Design review of the part built by this model. Coordinates are the model's own, in mm. Face numbers are marked on the shaded views. Round coordinates to 2 decimals unless told otherwise and drop trailing zeros. Write each loop counter-clockwise with the first axis right and the second up, starting at its lowest first coordinate (ties: lowest second). Pieces come first, ordered by that corner, then holes. Notation, with made-up numbers: M 72.25,-21.5 L 129.25,-21.5 A19 cw 129.25,-11.5 Z; hole C 36,5 d11. An arc over 180 degrees is marked long. Use CSV: the item, a comma, the result in double quotes.
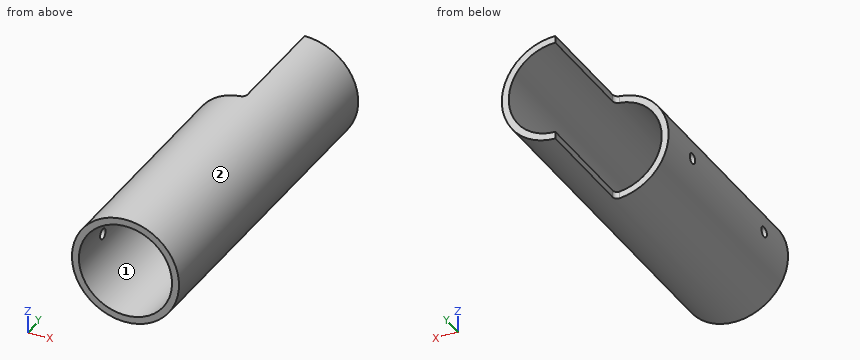
Autodesk Inventor part; units mm, degrees
ref_plane "YZ Plane" through (0, 0, 0) normal (1, 0, 0) x (0, 1, 0)
ref_plane "XZ Plane" through (0, 0, 0) normal (0, 1, 0) x (-1, 0, 0)
ref_plane "XY Plane" through (0, 0, 0) normal (0, 0, 1) x (1, 0, 0)
sketch "Sketch1" plane through (0, 0, 0) normal (0, 1, 0) x (-1, 0, 0)
  circle A0 centre (0, 0) radius 20
  circle A1 centre (0, 0) radius 23
  dimension "d0" = 40
  dimension "d1" = 3
extrude "Extrusion1" add sketch "Sketch1" along normal mid plane 150
sketch "Sketch2" plane through (0, 0, 0) normal (1, 0, 0) x (0, 1, 0)
  line L0 (-105, 0) -> (105, 0)
  line L1 (-75, 23) -> (-75, -23)
  point P0 (0, 0)
  point P1 (5, 0)
  point P2 (-55, 0)
  dimension "d4" = 60
  dimension "d5" = 20
hole "Hole1" at (0, 5, 0) at (0, -55, 0) direction (-1, 0, 0) diameter 4.5 end through all
sketch "Sketch3" plane through (0, 0, 0) normal (0, 0, 1) x (1, 0, 0)
  line L0 (23, 75) -> (-23, 75)
  line L1 (-23, -75) -> (-23, 75)
  line L2 (-23, 75) -> (0, 75)
  line L3 (0, 75) -> (0, 25)
  line L4 (0, 25) -> (-23, 25)
  line L5 (-23, 25) -> (-23, 75)
  point P0 (0, 0)
  dimension "d13" = 50
  dimension "d14" = 23
  dimension "d15" = 46
extrude "Extrusion2" cut sketch "Sketch3" along normal through all both and the other way through all
fillet "Fillet1" radius 2 2 edges at (0, 25, 21.5) (0, 25, -21.5)
equation "\"d14\" = 0.5 * d15"
properties part number "Pancake_Lower Pipe" material "PVC-Piping"
1) Add section B-B on x = 12. Write out the cut boundary in (y, z), then the cut area to 3 significant figures.
Answers:
outline,"M -75,-19.62 L 75,-19.62 L 75,-16 L -75,-16 Z; M -75,16 L 75,16 L 75,19.62 L -75,19.62 Z"
area,"1,090 mm²"
2) Add section D-D on y = -5. Write out the cut boundary in (x, z), then the cut area to 3 significant figures.
Answers:
outline,"C 0,0 d46; hole C 0,0 d40"
area,"405 mm²"
3) Wall thickness on line 1 along X through (y, z) = (11, 0); line 2 along X through (y, z) = (-37, 4): over which ranges is each line inside the solid? List them lowest first. Write a range as [from, to].
Answers:
line 1,"[-23, -20], [20, 23]"
line 2,"[-22.65, -19.6], [19.6, 22.65]"
4) Add section C-C on z = 11.5. Write out the cut boundary in (x, y).
Answers:
outline,"M -19.92,-75 L -16.36,-75 L -16.36,25 L -19.92,25 Z; M 16.36,-75 L 19.92,-75 L 19.92,75 L 16.36,75 Z"
5) The part is to be moulded in two halves that separate along X. For the marked faces 1 and 2, say which applies: released by +X, released by -X, zero draft, split by the parting line, or undercut.
Answers:
face 1,"undercut"
face 2,"split by the parting line"
6) For pin 1 Ø3.5 at (y, z) = (42.5, -21.5) entering from -X; pin 2 Ø5 at (y, z) = (-16, 0.5) entering from -X; pin 3 Ø10 at (x, y) = (-6, -5.5) entering from +Z; pin 4 Ø4 at (y, z) = (-54.5, 10) entering from -X, all flat-tipped, find the tip position at first contact; note any pin that passes through.
Answers:
pin 1,"x = 0"
pin 2,"x = -23"
pin 3,"z = 22.98"
pin 4,"x = -21.56"
7) Add section A-A on z = 0. Write out the cut boundary in (x, y).
Answers:
outline,"M -23,-75 L -20,-75 L -20,-57.25 L -23,-57.25 Z; M -23,-52.75 L -20,-52.75 L -20,2.75 L -23,2.75 Z; M -23,7.25 L -20,7.25 L -20,25 L -23,25 Z; M 20,-75 L 23,-75 L 23,75 L 20,75 Z"
